Autodesk Inventor part; units mm, degrees
ref_plane "YZ Plane" through (0, 0, 0) normal (1, 0, 0) x (0, 1, 0)
ref_plane "XZ Plane" through (0, 0, 0) normal (0, 1, 0) x (-1, 0, 0)
ref_plane "XY Plane" through (0, 0, 0) normal (0, 0, 1) x (1, 0, 0)
sketch "Sketch1" plane through (0, 0, 0) normal (0, 1, 0) x (-1, 0, 0)
  line L0 (0, 0) -> (26.416, 0)
  line L1 (26.416, 0) -> (26.416, -66.04)
  line L2 (26.416, -66.04) -> (0, -66.04)
  line L3 (0, -66.04) -> (0, 0)
  line L4 (29.591, -69.215) -> (29.591, 3.175)
  line L5 (29.591, 3.175) -> (-3.175, 3.175)
  line L6 (-3.175, 3.175) -> (-3.175, -69.215)
  line L7 (-3.175, -69.215) -> (29.591, -69.215)
  line L8 (13.208, -69.215) -> (18.208, -69.215)
  line L9 (18.208, -69.215) -> (18.208, -66.04)
  line L10 (18.208, -66.04) -> (13.208, -66.04)
  line L11 (13.208, -66.04) -> (13.208, -69.215)
  line L12 (13.208, -66.04) -> (8.208, -66.04)
  line L13 (8.208, -66.04) -> (8.208, -69.215)
  line L14 (8.208, -69.215) -> (13.208, -69.215)
  line L15 (13.208, -69.215) -> (13.208, -66.04)
  point P0 (18.208, -69.215)
  point P1 (8.208, -66.04)
  dimension "d0" = 26.416
  dimension "d1" = 66.04
  dimension "d2" = 3.175
  dimension "d3" = 5
  dimension "d4" = 5
extrude "Extrusion1" add sketch "Sketch1" along normal blind 7.62 contours L3 L2 L13 L7 L6 L5 L4 L9 L1 L0
sketch "Sketch2" plane through (0, 7.62, 0) normal (0, 1, 0) x (1, 0, 0)
  line L0 (-26.416, 0) -> (-26.416, 66.04)
  line L1 (-26.416, 0) -> (0, 0)
  line L2 (0, 0) -> (0, 66.04)
  line L3 (0, 66.04) -> (-26.416, 66.04)
  line L4 (-26.416, 66.04) -> (-26.416, 0)
  line L5 (-3.175, 3.175) -> (-23.241, 3.175)
  line L6 (-23.241, 3.175) -> (-23.241, 62.865)
  line L7 (-23.241, 62.865) -> (-3.175, 62.865)
  line L8 (-3.175, 62.865) -> (-3.175, 3.175)
  line L9 (-3.175, 3.175) -> (-6.175, 3.175)
  line L10 (-6.175, 3.175) -> (-6.175, 13.175)
  line L11 (-6.175, 13.175) -> (-3.175, 13.175)
  line L12 (-3.175, 13.175) -> (-3.175, 3.175)
  line L13 (-26.416, 66.04) -> (-18.208, 66.04)
  line L14 (0, 66.04) -> (0, 0)
  line L15 (-6.175, 13.175) -> (-6.675, 13.175)
  line L16 (-6.675, 13.175) -> (-6.675, 20.287)
  line L17 (-6.675, 20.287) -> (-6.175, 20.287)
  line L18 (-6.175, 20.287) -> (-6.175, 13.175)
  line L19 (-6.675, 20.287) -> (-23.6463, 20.287)
  line L20 (-23.6463, 20.287) -> (-23.6463, 23.8513)
  line L21 (-23.6463, 23.8513) -> (-6.675, 23.8513)
  line L22 (-6.675, 23.8513) -> (-6.675, 20.287)
  point P0 (-26.416, 66.04)
  dimension "d8" = 3.175
  dimension "d9" = 3
  dimension "d10" = 10
  dimension "d11" = 0.5
  dimension "d12" = 7.112
extrude "Extrusion2" add sketch "Sketch2" along normal blind 3.175 contours L0 L3 L2 L1 | L5 L6 L19 L16 L15 L10 | L11 L18 L17 L22 L21 L6 L7 L8 | L15 L16 L17 L18
sketch "Sketch3" plane through (0, 7.62, 0) normal (0, 1, 0) x (1, 0, 0)
  line L0 (-26.416, 66.04) -> (-18.208, 66.04)
  line L1 (-18.208, 66.04) -> (-18.208, 69.215)
  line L2 (-18.208, 69.215) -> (-29.591, 69.215)
  line L3 (-29.591, 69.215) -> (-29.591, -3.175)
  line L4 (-29.591, -3.175) -> (3.175, -3.175)
  line L5 (3.175, -3.175) -> (3.175, 69.215)
  line L6 (3.175, 69.215) -> (-8.208, 69.215)
  line L7 (-8.208, 69.215) -> (-8.208, 66.04)
  line L8 (-8.208, 66.04) -> (0, 66.04)
  line L9 (0, 66.04) -> (0, 0)
  line L10 (0, 0) -> (-26.416, 0)
  line L11 (-26.416, 0) -> (-26.416, 66.04)
extrude "Extrusion3" add sketch "Sketch3" along normal blind 3.175
fillet "Fillet1" radius 3.175 2 edges at (-18.208, 9.2075, -66.04) (-8.208, 9.2075, -66.04)
sketch "Sketch4" plane through (0, 0, 0) normal (0, -1, 0) x (1, 0, 0)
  line L0 (0, 0) -> (-26.416, 0)
  line L1 (-26.416, -66.04) -> (-18.208, -66.04)
  line L2 (0, 0) -> (-26.416, 0)
  line L3 (-26.416, 0) -> (-26.416, -66.04)
  line L4 (-26.416, -66.04) -> (0, -66.04)
  line L5 (0, -66.04) -> (0, 0)
  line L6 (0.254, 0.254) -> (-26.67, 0.254)
  line L7 (-26.67, 0.254) -> (-26.67, -66.294)
  line L8 (-26.67, -66.294) -> (0.254, -66.294)
  line L9 (0.254, -66.294) -> (0.254, 0.254)
  dimension "d18" = 0.254
extrude "Extrusion4" cut sketch "Sketch4" against normal up to surface (7.62 mm away) contours L5 L4 L1 L3 L0 | L9 L8 L7 L6
properties part number "RadioMountCover" material "Rubber, Silicone"
Input: part model. Units: mm. Frame: model coordinates. A direction names the side the tool comes from. Give positions to 0.01 mm unless a question says otherwise; leave off trailing zeros. Order: outer loops, then holes, each group sorted by start corner. A loop starts at its lowest first (then second) coordinate and runs counter-clockwise, first axis right, second up. Notation, with made-up numbers: (0.5, -1.75) - (37.5, -1.75) arc R22 cw to (37.5, 17.25) - close; hole circle Ø1 at (10, -31.75). An arc over 180 degrees is marked (long way). Answer as a JSON object with one key per item and string values. Group by question number.
Q1. Line query: probe 1 along Z at (x, y) = (-26, 1.25) (3 decimals); probe 2 along X at (y, z) = (4.75, -42.5) (3 decimals); probe 3 along Y at (x, z) = (-20, -44) (3 decimals). Output: solid intervals per line, ascending.
Q2. Cut plane D-D, the plane z = -37. Output: boundary loops of the cut face in (x, y) (3 decimals), then the cut area to 3 significant figures.
Q3. Cut plane B-B, the plane z = -11.5. Output: boundary loops of the cut face in (x, y) (3 decimals).
Q4. Mould query, pull axis X, two halves, no side actions, for faces 1 (the face through (3.175, 5, -33)), 2 (the face through (-9.16, 9.23, -66.95)), 3 (the face through (1, 0, -33)). Classes: pulls with the +X half, pulls with the -X half, needs draft (parallel to the pull), parting line crosses it, or undercut.
Q5. Cut plane A-A, the plane x = -4. Output: boundary loops of the cut face in (y, z) (3 decimals).
Q6. Set-up query: faces 4 (the face through (-8.208, 3, -68)), 5 (the face through (-15, 9, -23.851)), 6 (the face through (-22, 4, -66.294)). Return all of +Z, -Z, +X, -X, +Y, -Y with unobstructed straight access to the full face (end or side cutting, diameter ignored); none if empty.
Q7. First-contact query: pin 1 Ø13.5 at (x, z) = (-12.5, -50) entering from -Y; pin 2 Ø2.5 at (x, y) = (-13.5, 9) entering from -Z. Flat tips, straight axial feed; report the tip coordinate or a pass-through.
Q8. Cut plane C-C, the plane y = 2.25. Output: boundary loops of the cut face in (x, z) (3 decimals).
Results:
{
 "1": {"probe 1": "-69.215 to -66.294, 0.254 to 3.175", "probe 2": "-29.591 to -26.67, 0.254 to 3.175", "probe 3": "7.62 to 10.795"},
 "2": {"outline": "(-29.591, 0) - (-26.67, 0) - (-26.67, 7.62) - (0.254, 7.62) - (0.254, 0) - (3.175, 0) - (3.175, 10.795) - (-29.591, 10.795) - close", "area": "149 mm^2"},
 "3": {"outline": "(-29.591, 0) - (-26.67, 0) - (-26.67, 7.62) - (-6.175, 7.62) - (-6.175, 10.795) - (-29.591, 10.795) - close; (-3.175, 7.62) - (0.254, 7.62) - (0.254, 0) - (3.175, 0) - (3.175, 10.795) - (-3.175, 10.795) - close"},
 "4": {"face 1": "pulls with the +X half", "face 2": "undercut", "face 3": "needs draft"},
 "5": {"outline": "(0, -69.215) - (10.795, -69.215) - (10.795, -13.175) - (7.62, -13.175) - (7.62, -66.294) - (0, -66.294) - close; (0, 0.254) - (7.62, 0.254) - (7.62, -3.175) - (10.795, -3.175) - (10.795, 3.175) - (0, 3.175) - close"},
 "6": {"face 4": "-Z, -Y", "face 5": "+Y, -Y", "face 6": "-Y"},
 "7": {"pin 1": "y = 7.62", "pin 2": "z = -66.04"},
 "8": {"outline": "(-29.591, -69.215) - (-18.208, -69.215) - (-18.208, -66.294) - (-26.67, -66.294) - (-26.67, 0.254) - (0.254, 0.254) - (0.254, -66.294) - (-8.208, -66.294) - (-8.208, -69.215) - (3.175, -69.215) - (3.175, 3.175) - (-29.591, 3.175) - close"}
}
